from build123d import *

# Parameters (mm, degrees)
BASPROSKE_W         = 4
BASPROSKE_H         = 11
TOOTHCUT_DEPTH      = 17.062378404
TEETHCUTS_COUNT     = 20
TEETHCUTS_ANGLE     = 342
BORSKE_R            = 1
BORE_DEPTH          = 50.0000508
CUT_EXTRUDE_1_DEPTH = 10
EXTRUDE_1_REACH     = 39.733
SKETCH_3_W          = 4
SKETCH_3_H          = 4
FILLET_1_R          = 2
SKETCH_4_R          = 1.1
CUT_EXTRUDE_2_DEPTH = 10
EXTRUDE_START       = -4
SKETCH_5_R          = 1
EXTRUDE_2_DEPTH     = 4
EXTRUDE_3_DEPTH     = 1
EXTRUDE_START_2     = 4
EXTRUDE_4_DEPTH     = 4
SKETCH_8_R          = 3.6
CUT_EXTRUDE_3_DEPTH = 3.2
CUT_EXTRUDE_START   = -23.2
SKETCH_10_R         = 3.6
CUT_EXTRUDE_4_DEPTH = 23.2
SKETCH_11_R         = 3.6
EXTRUDE_5_DEPTH     = 1
CUT_EXTRUDE_START_2 = -1
SKETCH_12_R         = 3.6
CUT_EXTRUDE_5_DEPTH = 1
CUT_EXTRUDE_START_3 = -1.8
CUT_EXTRUDE_6_DEPTH = 1.8


with BuildPart() as part:
    # BasProSke → Base-Revolve (revolve)
    with BuildSketch(Plane(origin=(0, 0, 0), x_dir=(1, 0, 0), z_dir=(0, 1, 0)), mode=Mode.PRIVATE) as base_revolve_sk:
        with Locations((2, 5.5)):
            Rectangle(BASPROSKE_W, BASPROSKE_H)
    revolve(base_revolve_sk.sketch.rotate(Axis((-10, 0, 0), (1, 0, 0)), 180), axis=Axis((-10, 0, 0), (1, 0, 0)))

    # TooCutSke → ToothCut (cut, through all)
    with BuildSketch(Plane(origin=(0, 0, 0), x_dir=(0, 0, -1), z_dir=(1, 0, 0))):
        with BuildLine():
            ThreePointArc((0.499924007, 8.734705318), (0, 8.749), (-0.499924007, 8.734705318))
            ThreePointArc((-0.499924007, 8.734705318), (-0.824302243, 9.905497836), (-1.485192705, 10.924909509))
            ThreePointArc((-1.485192705, 10.924909509), (0, 11.0254), (1.485192705, 10.924909509))
            ThreePointArc((1.485192705, 10.924909509), (0.824302243, 9.905497836), (0.499924007, 8.734705318))
        make_face()
    toothcut = extrude(amount=TOOTHCUT_DEPTH, mode=Mode.SUBTRACT)

    # TeethCuts: ToothCut ×20 about axis
    teethcuts_axis = Axis((-10, 0, 0), (1, 0, 0))
    for i in range(1, TEETHCUTS_COUNT):
        add(toothcut.rotate(teethcuts_axis, i * TEETHCUTS_ANGLE / (TEETHCUTS_COUNT - 1)), mode=Mode.SUBTRACT)

    # BorSke → Bore (cut, symmetric)
    with BuildSketch(Plane(origin=(0, 0, 0), x_dir=(0, 0, -1), z_dir=(1, 0, 0))):
        with Locations(Location((0, 0, 0), (0, 0, 180))):
            Circle(BORSKE_R)
    extrude(amount=BORE_DEPTH, both=True, mode=Mode.SUBTRACT)

    # 草图1 → 切除-拉伸1 (cut)
    with BuildSketch(Plane(origin=(4, 0, 0), x_dir=(0, 0, -1), z_dir=(1, 0, 0))):
        with BuildLine():
            Line((0, 12.401538845), (0, 2.5))
            ThreePointArc((0, 2.5), (1.767766953, 1.767766953), (2.5, 0))
            ThreePointArc((2.5, 0), (1.767766953, -1.767766953), (0, -2.5))
            Line((0, -2.5), (0, -15.030002789))
            Line((0, -15.030002789), (15.193341894, -15.030002789))
            Line((15.193341894, -15.030002789), (15.193341894, 12.401538845))
            Line((15.193341894, 12.401538845), (0, 12.401538845))
        make_face()
    extrude(amount=-CUT_EXTRUDE_1_DEPTH, mode=Mode.SUBTRACT)

    # 草图3 → 凸台-拉伸1 (add, up to next)
    with BuildSketch(Plane(origin=(0, -25, 0), x_dir=(1, 0, 0), z_dir=(0, 1, 0)), mode=Mode.PRIVATE) as extrude_1_sk1:
        with Locations((2, 0.024348859)):
            Rectangle(SKETCH_3_W, SKETCH_3_H)
    extrude_1_tool1 = extrude(extrude_1_sk1.sketch, amount=EXTRUDE_1_REACH, mode=Mode.PRIVATE) - part.part
    add(extrude_1_tool1.solids().sort_by_distance((2, -25, -0.024349))[0])

    # 圆角1
    fillet_1_edges = [part.edges().sort_by_distance(p)[0] for p in [
        (2, -25, 1.975651141),
        (2, -25, -2.024348859),
    ]]
    fillet(fillet_1_edges, radius=FILLET_1_R - 0.0001)  # a hair under: the kernel refuses the full size

    # 草图4 → 切除-拉伸2 (cut)
    with BuildSketch(Plane(origin=(4, 0, 0), x_dir=(0, 0, -1), z_dir=(1, 0, 0))):
        with Locations((0.024348859, -23)):
            Circle(SKETCH_4_R)
    extrude(amount=-CUT_EXTRUDE_2_DEPTH, mode=Mode.SUBTRACT)

    # 草图5 → 凸台-拉伸2 (add)
    with BuildSketch(Plane.ZY.offset(EXTRUDE_START)):
        Circle(SKETCH_5_R)
    extrude(amount=EXTRUDE_2_DEPTH)

    # 草图6 → 凸台-拉伸3 (add)
    with BuildSketch(Plane.ZY):
        with BuildLine():
            Line((0, 5), (0, 2.5))
            ThreePointArc((0, 2.5), (-2.226817699, 1.136346309), (-2.024348859, -1.466973653))
            Line((-2.024348859, -1.466973653), (-2.024348859, -4.571871794))
            ThreePointArc((-2.024348859, -4.571871794), (2.727476463, -4.19056943), (5, 0))
            ThreePointArc((5, 0), (3.535533906, 3.535533906), (0, 5))
        make_face()
        with BuildLine():
            ThreePointArc((-2.024348859, -1.466973653), (-2.226817699, 1.136346309), (0, 2.5))
            Line((0, 2.5), (0, 5))
            ThreePointArc((0, 5), (-4.891797163, 1.034562959), (-2.024348859, -4.571871794))
            Line((-2.024348859, -4.571871794), (-2.024348859, -1.466973653))
        make_face()
        with BuildLine():
            Line((0, 5), (0, 2.5))
            ThreePointArc((0, 2.5), (-2.226817699, 1.136346309), (-2.024348859, -1.466973653))
            Line((-2.024348859, -1.466973653), (-2.024348859, -4.571871794))
            ThreePointArc((-2.024348859, -4.571871794), (2.727476463, -4.19056943), (5, 0))
            ThreePointArc((5, 0), (3.535533906, 3.535533906), (0, 5))
        make_face()
        with BuildLine():
            ThreePointArc((-2.024348859, -1.466973653), (-2.226817699, 1.136346309), (0, 2.5))
            Line((0, 2.5), (0, 5))
            ThreePointArc((0, 5), (-4.891797163, 1.034562959), (-2.024348859, -4.571871794))
            Line((-2.024348859, -4.571871794), (-2.024348859, -1.466973653))
        make_face()
    extrude(amount=EXTRUDE_3_DEPTH)

    # 草图7 → 凸台-拉伸4 (add)
    with BuildSketch(Plane(origin=(0, 0, 0), x_dir=(0, 0, -1), z_dir=(1, 0, 0)).offset(EXTRUDE_START_2)):
        with BuildLine():
            Line((0, 5), (0, 2.5))
            ThreePointArc((0, 2.5), (2.226817699, 1.136346309), (2.024348859, -1.466973653))
            Line((2.024348859, -1.466973653), (2.024348859, -4.571871794))
            ThreePointArc((2.024348859, -4.571871794), (4.891797163, 1.034562959), (0, 5))
        make_face()
    extrude(amount=-EXTRUDE_4_DEPTH)

    # 草图8 → 切除-拉伸3 (cut)
    with BuildSketch(Plane(origin=(4, 0, 0), x_dir=(0, 0, -1), z_dir=(1, 0, 0))):
        Circle(SKETCH_8_R)
    extrude(amount=-CUT_EXTRUDE_3_DEPTH, mode=Mode.SUBTRACT)

    # 草图10 → 切除-拉伸4 (cut)
    with BuildSketch(Plane.ZY.offset(1).offset(CUT_EXTRUDE_START)):
        with Locations(Location((0, 0, 0), (0, 0, 180))):
            Circle(SKETCH_10_R)
    extrude(amount=CUT_EXTRUDE_4_DEPTH, mode=Mode.SUBTRACT)

    # 草图11 → 凸台-拉伸5 (add)
    with BuildSketch(Plane(origin=(4, 0, 0), x_dir=(0, 0, -1), z_dir=(1, 0, 0))):
        Circle(SKETCH_11_R)
    extrude(amount=-EXTRUDE_5_DEPTH)

    # 草图12 → 切除-拉伸5 (cut)
    with BuildSketch(Plane.ZY.offset(-3).offset(CUT_EXTRUDE_START_2)):
        Circle(SKETCH_12_R)
    extrude(amount=CUT_EXTRUDE_5_DEPTH, mode=Mode.SUBTRACT)

    # 草图13 → 切除-拉伸6 (cut)
    with BuildSketch(Plane.ZY.offset(1).offset(CUT_EXTRUDE_START_3)):
        with BuildLine():
            Line((6, 2.564298292), (2.227527106, 2.828095294))
            ThreePointArc((2.227527106, 2.828095294), (3.6, 0), (2.227527106, -2.828095294))
            Line((2.227527106, -2.828095294), (6, -2.564298292))
            Line((6, -2.564298292), (6, 2.564298292))
        make_face()
    extrude(amount=CUT_EXTRUDE_6_DEPTH, mode=Mode.SUBTRACT)


solid = part.part
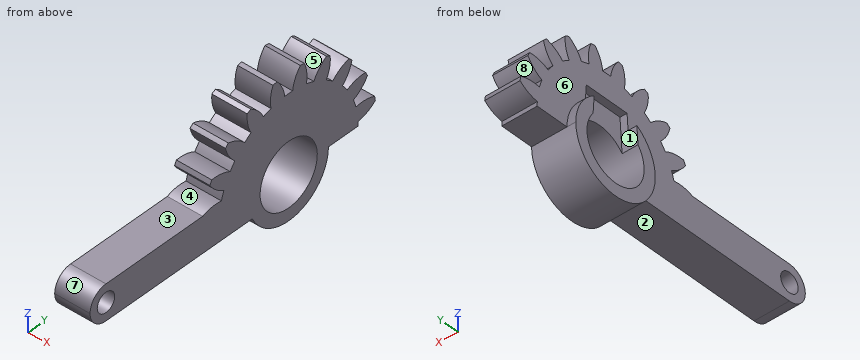
Source: CAD feature listing. Evaluate the final solid. Frame: model axes, mm. Face numbers are marked on the shaded views. A direction names the side the tool comes from. Round coordinates to 2 decimals unless told otherwise and drop trailing zeros. Loops run counter-clockwise (first coordinate to the right, second up) from the corner with the lowest first, then second, coordinate; pieces in that order, holes last. Notation, with made-up numbers: M 47,10.5 L 90,10.5 A32 ccw 90,40.5 Z; hole C -11,-21.75 d2. An arc over 180 degrees is marked long. Return JSON: item names as keys, results as strings. Group by question number.
1. Section query B-B on x = 3.55. State how many separate pieces and enclosed holes the cut face has, and give its area (3 significant figures).
2. Section query A-A on y = -18.5. Output: boundary loops of the cut face in (x, z), and give its area (3 significant figures).
3. Material intervals for line 1 along Z through (x, y) = (2.3, 0); line 2 along Y through (x, z) = (1.55, 7.5); line 3 along Y through (x, z) = (2.15, -0.25), sorted ascending. Write a range as from..to.
4. Section query D-D on y = -4. Output: boundary loops of the cut face in (x, z), and give its area (3 significant figures).
5. Mould query, pull axis Z, two halves, no side actions, for the marked faces 6, 7 and 8. Classes: released by +Z, released by -Z, zero draft, split by the parting line, or undercut.
6. Pin query (flat end, axial travel): pin 1 (1.9 mm diameter, centred on x = 2.5, y = 6, fed in from -Z); pin 2 (1.2 mm diameter, centred on x = 2.5, y = -17, fed in from +Z); pin 3 (1 mm diameter, centred on y = -5.5, z = -3, fed in from +X); pin 4 (1.9 mm diameter, centred on y = 0.5, z = 5, fed in from -X). Return the tip coordinate at first contact, or that it passes through.
7. Reachability of the marked faces 1, 2, 3, 4 and 5 from +Z, -Z, +X, -X, +Y, -Y: full face, straight path, thin tool, end or side. Return the list, or none.
Checks:
{
 "1": {"separate pieces": "1", "enclosed holes": "2", "area": "215 mm²"},
 "2": {"outline": "M 0,-2.02 L 4,-2.02 L 4,1.98 L 0,1.98 Z", "area": "16.0 mm²"},
 "3": {"line 1": "z = -5..-3.6, 3.6..8.75", "line 2": "y = -7.94..-6.44, -4.8..4.8, 6.44..7.94", "line 3": "y = -24.99..-24.08, -21.92..-3.59, 3.59..4.99"},
 "4": {"outline": "M -1,-3 L 4,-3 L 4,9.33 L 0,9.33 L 0,3 L -1,3 Z", "area": "55.3 mm²"},
 "5": {"face 6": "zero draft", "face 7": "released by +Z", "face 8": "undercut"},
 "6": {"pin 1": "stops at z = 0", "pin 2": "stops at z = 1.98", "pin 3": "passes through", "pin 4": "stops at x = 0.8"},
 "7": {"face 1": "-X", "face 2": "-Z, +X, -X, -Y", "face 3": "+Z, +X, -X, -Y", "face 4": "+X, -X", "face 5": "+Z, +X, -X"}
}
